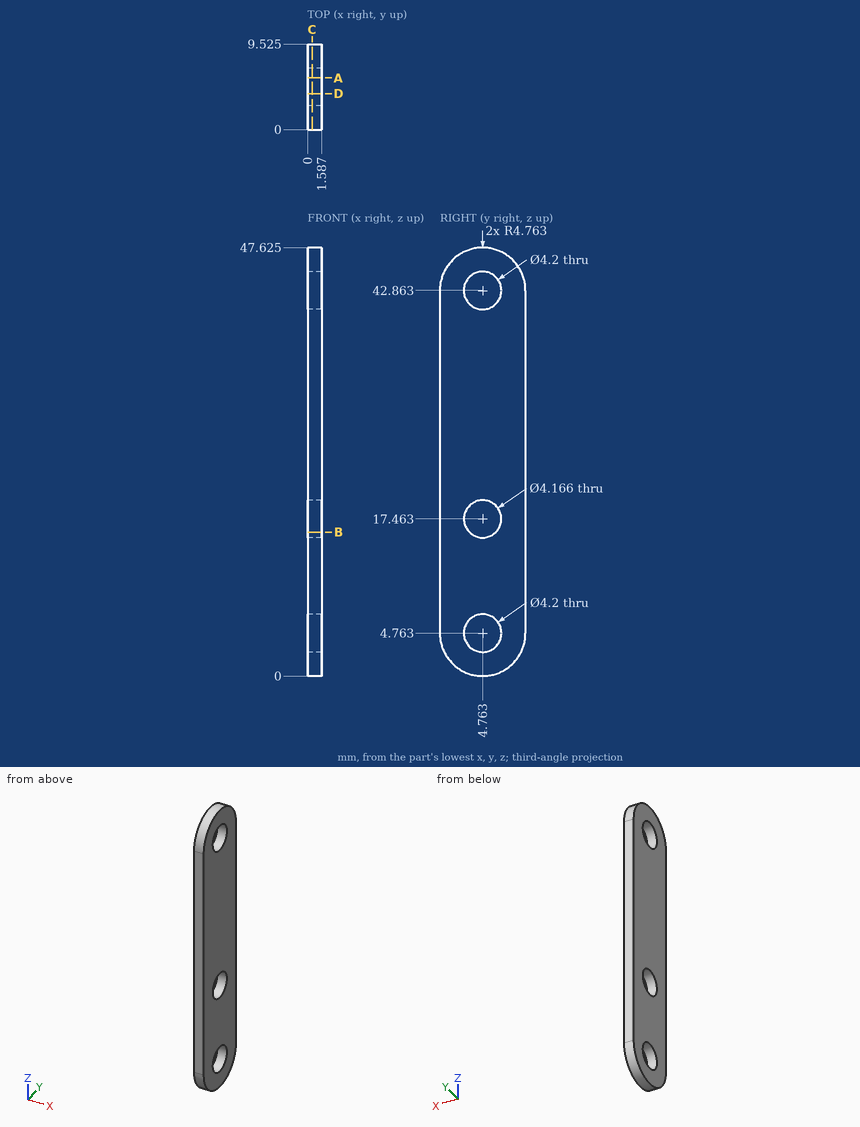
Answer from the drawing. Dimensions are ordinates in mm from the lowest x, y and z of the part. Round coordinates to 2 decimals unless told otherwise and drop trailing zeros. Write each loop counter-clockwise with the first axis right and the second up, starting at its lowest first coordinate (ties: lowest second). Pieces come first, ordered by that corner, then holes.
1. The part is cut by section D-D, the plane y = 4. Determine the outline of the cut face in (x, z) (1 decimal).
2. The part is cut by section C-C, the plane x = 0.5. Determine the outline of the cut face in (y, z) (1 decimal), then the cut area to 3 significant figures.
3. Given pin 1 Ø4 at (y, z) = (4.76, 42.86) entering from -X; pin 2 Ø5 at (y, z) = (4.76, 17.46) entering from +X, each flat-ended and moving along its own axis, determine where each tip first touches the part or whether it passes through.
4. The part is cut by section B-B, the plane z = 16. Determine the outline of the cut face in (x, y) (1 decimal).
5. The part is cut by section A-A, the plane y = 5.75. Determine the outline of the cut face in (x, z) (1 decimal).
6. Straight lines are drawn through the part: L1, parallel to Z at x = 1.45, y = 4.75 (1 decimal); L2, parallel to Z at x = 0.15, y = 4 (1 decimal); L3, parallel to Y at x = 0.3, z = 5.5 (1 decimal). For each, find the intervals that lie inside material, in ascending order.
Values:
1. outline: (0, 0.1) - (1.6, 0.1) - (1.6, 2.8) - (0, 2.8) - close; (0, 6.7) - (1.6, 6.7) - (1.6, 15.5) - (0, 15.5) - close; (0, 19.4) - (1.6, 19.4) - (1.6, 40.9) - (0, 40.9) - close; (0, 44.8) - (1.6, 44.8) - (1.6, 47.6) - (0, 47.6) - close
2. outline: (0, 4.8) arc R4.8 ccw to (9.5, 4.8) - (9.5, 42.9) arc R4.8 ccw to (0, 42.9) - close; hole circle Ø4.2 at (4.8, 4.8); hole circle Ø4.2 at (4.8, 17.5); hole circle Ø4.2 at (4.8, 42.9)
2. area: 393 mm2
3. pin 1: passes through
3. pin 2: stops at x = 1.59
4. outline: (0, 0) - (1.6, 0) - (1.6, 3.3) - (0, 3.3) - close; (0, 6.2) - (1.6, 6.2) - (1.6, 9.5) - (0, 9.5) - close
5. outline: (0, 0.1) - (1.6, 0.1) - (1.6, 2.9) - (0, 2.9) - close; (0, 6.6) - (1.6, 6.6) - (1.6, 15.6) - (0, 15.6) - close; (0, 19.3) - (1.6, 19.3) - (1.6, 41) - (0, 41) - close; (0, 44.7) - (1.6, 44.7) - (1.6, 47.5) - (0, 47.5) - close
6. L1: z = 0 to 2.7, 6.9 to 15.4, 19.5 to 40.8, 45 to 47.6
6. L2: z = 0.1 to 2.8, 6.7 to 15.5, 19.4 to 40.9, 44.8 to 47.6
6. L3: y = 0 to 2.8, 6.7 to 9.5
